Here's how the part is built. I have some questions about the finished solid (model axes, mm). Give positions to 0.01 mm unless a question says otherwise; leave off trailing zeros. Order: outer loops, then holes, each group sorted by start corner. A loop starts at its lowest first (then second) coordinate and runs counter-clockwise, first axis right, second up. Notation, with made-up numbers: (81, -26.75) -> (131, -26.75) arc R13 cw to (131, -13.75) -> close; hole circle Ø7 at (4.5, 25). An arc over 180 degrees is marked (long way). Write each question's results on one line, items separated by ' | '. Start each with the question number.
Q1. I need wall thicknesses on line 1 along X through (y, z) = (2.25, -10); line 2 along Z through (x, y) = (32.5, 1.4); line 3 along X through (y, z) = (0.4, -9). Which ranges of each line are inside material? Lowest first, please. Write a range as [from, to].
Q2. I'm going to push a flat-ended pin straight in: pin 1 (3 mm diameter, centred on x = -32.5, z = 10, fed in from -Y). Where does the tip first touch, or does it pass through?
Q3. Imagine slicing it at B-B, the plane x = -32.5. Please give me the cut outline in (y, z), then the cut area to 3 significant figures.
Q4. Imagine slicing it at C-C, the plane y = 1.85. Please give me the cut outline in (x, z).
Q5. Imagine slicing it at A-A, the plane z = 10. Please give me the cut outline in (x, y), then the cut area to 3 significant figures.
Q6. Thinking about a two-plate mould opening in Z: for faces 1 (the face through (30, 2, -10)), 2 (the face through (-30, 2, -10)), 3 (the face through (-1, 5, 0)), 4 (the face through (-57, 3, 19)), which applies, pulls with the +Z half, pulls with the -Z half, needs draft (parallel to the pull), parting line crosses it, or undercut?
```python
from build123d import *

# Parameters (mm, degrees)
SKETCH1_W           = 115
SKETCH1_H           = 40
SKETCH1_R           = 2.5
BOSS_EXTRUDE1_DEPTH = 5
FILLET1_R           = 2.5
CHAMFER1_SIZE       = 1


with BuildPart() as part:
    # Sketch1 → Boss-Extrude1 (new body)
    with BuildSketch(Plane(origin=(0, 0, 0), x_dir=(1, 0, 0), z_dir=(0, 1, 0))):
        Rectangle(SKETCH1_W, SKETCH1_H)
        with Locations(Location((-32.5, 10, 0), (0, 0, 270))):
            Circle(SKETCH1_R, mode=Mode.SUBTRACT)
        with Locations(Location((-32.5, -10, 0), (0, 0, 270))):
            Circle(SKETCH1_R, mode=Mode.SUBTRACT)
        with Locations(Location((32.5, -10, 0), (0, 0, 90))):
            Circle(SKETCH1_R, mode=Mode.SUBTRACT)
        with Locations(Location((32.5, 10, 0), (0, 0, 90))):
            Circle(SKETCH1_R, mode=Mode.SUBTRACT)
    extrude(amount=BOSS_EXTRUDE1_DEPTH)

    # Fillet1
    fillet1_edges = [part.edges().sort_by_distance(p)[0] for p in [
        (57.5, 2.5, 20),
        (-57.5, 2.5, 20),
        (-57.5, 2.5, -20),
        (57.5, 2.5, -20),
    ]]
    fillet(fillet1_edges, radius=FILLET1_R)

    # Chamfer1
    chamfer1_edges = [part.edges().sort_by_distance(p)[0] for p in [
        (-32.5, 5, -12.5),
        (-32.5, 5, 7.5),
        (32.5, 5, 12.5),
        (32.5, 5, -7.5),
    ]]
    chamfer(chamfer1_edges, length=CHAMFER1_SIZE)


solid = part.part
```
Geometry check:
1) line 1: [-57.5, -35], [-30, 30], [35, 57.5] | line 2: [-20, -12.5], [-7.5, 7.5], [12.5, 20] | line 3: [-57.5, -34.79], [-30.21, 30.21], [34.79, 57.5]
2) pin 1: through
3) outline: (0, -20) -> (5, -20) -> (5, -13.5) -> (4, -12.5) -> (0, -12.5) -> close; (0, -7.5) -> (4, -7.5) -> (5, -6.5) -> (5, 6.5) -> (4, 7.5) -> (0, 7.5) -> close; (0, 12.5) -> (4, 12.5) -> (5, 13.5) -> (5, 20) -> (0, 20) -> close | area: 148 mm²
4) outline: (-57.5, -17.5) arc R2.5 ccw to (-55, -20) -> (55, -20) arc R2.5 ccw to (57.5, -17.5) -> (57.5, 17.5) arc R2.5 ccw to (55, 20) -> (-55, 20) arc R2.5 ccw to (-57.5, 17.5) -> close; hole circle Ø5 at (-32.5, -10); hole circle Ø5 at (-32.5, 10); hole circle Ø5 at (32.5, -10); hole circle Ø5 at (32.5, 10)
5) outline: (-57.5, 0) -> (-35, 0) -> (-35, 4) -> (-36, 5) -> (-57.5, 5) -> close; (-30, 0) -> (30, 0) -> (30, 4) -> (29, 5) -> (-29, 5) -> (-30, 4) -> close; (35, 0) -> (57.5, 0) -> (57.5, 5) -> (36, 5) -> (35, 4) -> close | area: 523 mm²
6) face 1: undercut | face 2: undercut | face 3: needs draft | face 4: pulls with the +Z half
